Geometry: final body of the model. Coordinates: model frame, mm. A direction names the side the tool comes from. Give positions to 0.01 mm unless a question says otherwise; leave off trailing zeros. Write each loop counter-clockwise with the first axis right and the second up, starting at its lowest first coordinate (ties: lowest second). Pieces come first, ordered by that corner, then holes. Notation, with made-up numbers: M 81,-39.5 L 135,-39.5 A14 cw 135,-32.5 Z; hole C 19,-0.75 d5. An arc over 180 degrees is marked long. Use a Markdown table: item, result. Add a question column.
(1) Cut plane B-B (y = 10). Output: boundary loops of the cut face in (x, z), plus the area to 3 significant figures.
(2) Reachability of faces 1 (the flat face through (25, 17, 15)), 2 (the flat face through (46, 15.9, 9)) from +Z, -Z, +X, -X, +Y, -Y: full face, straight path, thin tool, end or side. Return the list, or none.
(3) Draft query along X for faces 3 (the cylindrical face through (62, 10, 7)), 4 (the cylindrical face through (-10, 10, 7)), 5 (the flat face through (43.5, 10, 9)). Return one class per face: released by +X, released by -X, zero draft, split by the parting line, or undercut.
(4) Pin query (flat end, axial travel): pin 1 Ø4 at (y, z) = (11, 4) entering from -X; pin 2 Ø3 at (y, z) = (2, 7) entering from -X; pin 3 Ø1.5 at (x, y) = (6.5, 7.5) entering from +Z. Return the tip coordinate at first contact, or that it passes through.
(5) Cut plane A-A (z = 5.5). Output: boundary loops of the cut face in (x, y), plus the area to 3 significant figures.
(6) Cut plane D-D (y = 14). Output: boundary loops of the cut face in (x, z), plus the area to 3 significant figures.
(7) Cut plane C-C (z = 2.5). Output: boundary loops of the cut face in (x, y).
(8) Material intervals for L1, parallel to X at y = 11.75, z = 4.25; L2, parallel to X at y = 6.5, z = 5.25; L3, parallel to Y at x = 25, z = 12.25, sorted ascending.
```python
from build123d import *

# Parameters (mm, degrees)
BOX003_W          = 4.9
BOX003_H          = 12.4
BOX003_DEPTH      = 20
BOX002_W          = 4.9
BOX002_H          = 12.4
BOX002_DEPTH      = 20
BOX001_W          = 4.9
BOX001_H          = 12.4
BOX001_DEPTH      = 20
CYLINDER_R        = 10
CYLINDER_DEPTH    = 15
CYLINDER001_R     = 10
CYLINDER001_DEPTH = 15
BOX_W             = 52
BOX_H             = 20
BOX_DEPTH         = 15


with BuildPart() as slot003:
    # Box003 → Box003 (new body)
    with BuildSketch(Plane(origin=(43.5, 3.5, 4), x_dir=(1, 0, 0), z_dir=(0, 0, 1))):
        with Locations((2.45, 6.2)):
            Rectangle(BOX003_W, BOX003_H)
    extrude(amount=BOX003_DEPTH)


with BuildPart() as slot002:
    # Box002 → Box002 (new body)
    with BuildSketch(Plane(origin=(23.5, 3.5, 4), x_dir=(1, 0, 0), z_dir=(0, 0, 1))):
        with Locations((2.45, 6.2)):
            Rectangle(BOX002_W, BOX002_H)
    extrude(amount=BOX002_DEPTH)


with BuildPart() as slots:
    # Box001 → Box001 (new body)
    with BuildSketch(Plane(origin=(3.5, 3.5, 4), x_dir=(1, 0, 0), z_dir=(0, 0, 1))):
        with Locations((2.45, 6.2)):
            Rectangle(BOX001_W, BOX001_H)
    extrude(amount=BOX001_DEPTH)

    # Fusion: union slot003, slot002
    add(slot003.part)
    add(slot002.part)


with BuildPart() as cilindro:
    # Cylinder → Cylinder (new body)
    with BuildSketch(Plane(origin=(0, 10, 0), x_dir=(1, 0, 0), z_dir=(0, 0, 1))):
        Circle(CYLINDER_R)
    extrude(amount=CYLINDER_DEPTH)


with BuildPart() as cilindro001:
    # Cylinder001 → Cylinder001 (new body)
    with BuildSketch(Plane(origin=(52, 10, 0), x_dir=(1, 0, 0), z_dir=(0, 0, 1))):
        Circle(CYLINDER001_R)
    extrude(amount=CYLINDER001_DEPTH)


with BuildPart() as cut:
    # Box → Box (new body)
    with BuildSketch(Plane.XY):
        with Locations((26, 10)):
            Rectangle(BOX_W, BOX_H)
    extrude(amount=BOX_DEPTH)

    # Fusion001: union Cilindro, Cilindro001
    add(cilindro.part)
    add(cilindro001.part)

    # Cut: cut slots
    add(slots.part, mode=Mode.SUBTRACT)


solid = cut.part
```
Answer list:
| question | item | result |
|---|---|---|
| 1 | outline | M -10,0 L 62,0 L 62,15 L 48.4,15 L 48.4,4 L 43.5,4 L 43.5,15 L 28.4,15 L 28.4,4 L 23.5,4 L 23.5,15 L 8.4,15 L 8.4,4 L 3.5,4 L 3.5,15 L -10,15 Z |
| 1 | area | 918 mm² |
| 2 | face 1 | +Z, +X, -X, +Y, -Y |
| 2 | face 2 | +Z |
| 3 | face 3 | released by +X |
| 3 | face 4 | released by -X |
| 3 | face 5 | undercut |
| 4 | pin 1 | x = -10 |
| 4 | pin 2 | x = -7.6 |
| 4 | pin 3 | z = 4 |
| 5 | outline | M 0,0 L 52,0 A10 ccw 52,20 L 0,20 A10 ccw Z; hole M 3.5,3.5 L 8.4,3.5 L 8.4,15.9 L 3.5,15.9 Z; hole M 23.5,3.5 L 28.4,3.5 L 28.4,15.9 L 23.5,15.9 Z; hole M 43.5,3.5 L 48.4,3.5 L 48.4,15.9 L 43.5,15.9 Z |
| 5 | area | 1,170 mm² |
| 6 | outline | M -9.17,0 L 61.17,0 L 61.17,15 L 48.4,15 L 48.4,4 L 43.5,4 L 43.5,15 L 28.4,15 L 28.4,4 L 23.5,4 L 23.5,15 L 8.4,15 L 8.4,4 L 3.5,4 L 3.5,15 L -9.17,15 Z |
| 6 | area | 893 mm² |
| 7 | outline | M 0,0 L 52,0 A10 ccw 52,20 L 0,20 A10 ccw Z |
| 8 | L1 | -9.85 to 3.5, 8.4 to 23.5, 28.4 to 43.5, 48.4 to 61.85 |
| 8 | L2 | -9.37 to 3.5, 8.4 to 23.5, 28.4 to 43.5, 48.4 to 61.37 |
| 8 | L3 | 0 to 3.5, 15.9 to 20 |
